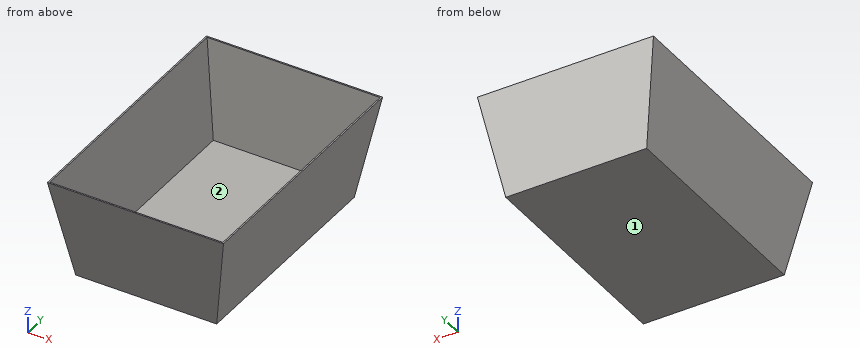
```python
from build123d import *

# Parameters (mm, degrees)
F0_W     = 431.8
F0_H     = 685.8
F1_DEPTH = 304.8
F1_TAPER = -10
F3_W     = 431.8
F3_H     = 685.8
F4_DEPTH = 279.4
F4_TAPER = -10


with BuildPart() as f1:
    # F0 (on Top) → F1 (new body)
    with BuildSketch(Plane.XY):
        Rectangle(F0_W, F0_H)
    extrude(amount=F1_DEPTH, taper=F1_TAPER)

    # F3 (on offset) → F4 (cut)
    with BuildSketch(Plane.XY.offset(25.4)):
        Rectangle(F3_W, F3_H)
    extrude(amount=F4_DEPTH, taper=F4_TAPER, mode=Mode.SUBTRACT)


solid = f1.part
```
Work out the finished part from the listing and answer in its coordinate system (mm). Face numbers are marked on the shaded views. Give positions to 0.01 mm unless a question says otherwise; leave off trailing zeros. Write item = value, one per line. Start each with the question number.
(1) The mould has two halves that part along Y. Classify the marked faces 1 and 2: +Y half, -Y half, draft (parallel to the pull), parting line (faces both ways), or undercut.
(2) Find the intervals of material crossed by probe 1 along Z at (x, y) = (123.5, 298); probe 2 along Y at (x, z) = (188, 82); probe 3 along X at (y, z) = (-206, 32), in increasing order. Write a range as from..to.
(3) Given pin 1 Ø6 at (x, z) = (137, 156.5) entering from -Y; pin 2 Ø4 at (x, z) = (120, 74) entering from -Y; pin 3 Ø5 at (x, z) = (-38, 73) entering from +Y, each flat-ended and moving along its own axis, determine where each tip first touches the part or whether it passes through.
From the geometry:
q1.face_1 = draft
q1.face_2 = undercut
q2.probe_1 = 0..25.4
q2.probe_2 = -357.36..-352.88, 352.88..357.36
q2.probe_3 = -221.54..-217.06, 217.06..221.54
q3.pin_1 = -371.02
q3.pin_2 = -356.3
q3.pin_3 = 356.21
